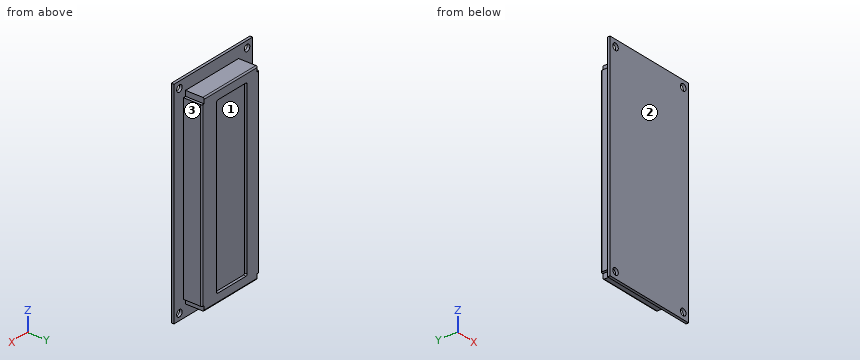
Autodesk Inventor part; units mm, degrees
ref_plane "YZ Plane" through (0, 0, 0) normal (1, 0, 0) x (0, 1, 0)
ref_plane "XZ Plane" through (0, 0, 0) normal (0, 1, 0) x (-1, 0, 0)
ref_plane "XY Plane" through (0, 0, 0) normal (0, 0, 1) x (1, 0, 0)
sketch "Sketch1" plane through (0, 0, 0) normal (0, 1, 0) x (-1, 0, 0)
  line L0 (-18, 40) -> (-18, -40)
  line L1 (-18, -40) -> (18, -40)
  line L2 (18, -40) -> (18, 40)
  line L3 (18, 40) -> (-18, 40)
  line L4 (-18, 40) -> (18, -40) construction
  line L5 (-18, -40) -> (18, 40) construction
  line L6 (18, 40) -> (-0.55, 40)
  line L7 (18, 40) -> (15.5, 40)
  line L8 (15.5, 40) -> (15.5, 37.5)
  circle A0 centre (15.5, 37.5) radius 1.25
  line L9 (15.5, 37.5) -> (-15.5, 37.5)
  line L10 (-15.5, 37.5) -> (-15.5, -37.5)
  line L11 (-15.5, -37.5) -> (15.5, -37.5)
  circle A1 centre (-15.5, 37.5) radius 1.25
  circle A2 centre (-15.5, -37.5) radius 1.25
  circle A3 centre (15.5, -37.5) radius 1.25
  point P0 (0, 0)
  dimension "d0" = 80
  dimension "d1" = 36
  dimension "d2" = 18.55
  dimension "d25" = 2.5
  dimension "d26" = 2.5
  dimension "d27" = 2.5
  dimension "d28" = 31
  dimension "d29" = 75
  dimension "d30" = 31
  dimension "d31" = 2.5
  dimension "d32" = 2.5
  dimension "d33" = 2.5
extrude "Extrusion1" add sketch "Sketch1" along normal blind 1 contours A3 | A2 L11 L10 | L10 L11 A2 | A1 L10 L9 | L9 L10 A1 | A0 L9 L8 | L8 L9 A0 | L3 L2 L1 L0
sketch "Sketch2" plane through (0, 1, 0) normal (0, 1, 0) x (1, 0, 0)
  line L0 (18, -40) -> (18, 40)
  line L1 (18, 40) -> (-18, 40)
  line L2 (-18, 40) -> (-18, -40)
  line L3 (-18, -40) -> (18, -40)
  line L4 (-18, -40) -> (0.55, -40)
  line L5 (-18, -40) -> (18, -40)
  line L6 (-11.6, -35.65) -> (-11.6, -33.65)
  line L7 (-11.6, -33.65) -> (-12.6, -33.65)
  line L8 (12.7, -35.65) -> (12.7, -33.65)
  line L9 (12.7, -33.65) -> (13.7, -33.65)
  line L10 (12.7, 35.65) -> (12.7, 33.65)
  line L11 (12.7, 33.65) -> (13.7, 33.65)
  line L12 (-11.6, 35.65) -> (-11.6, 33.65)
  line L13 (-11.6, 33.65) -> (-12.6, 33.65)
  line L14 (-11.6, -35.65) -> (12.7, -35.65)
  line L15 (13.7, -33.65) -> (13.7, 33.65)
  line L16 (12.7, 35.65) -> (-11.6, 35.65)
  line L17 (-12.6, 33.65) -> (-12.6, -33.65)
  point P0 (0, 0)
  dimension "d10" = 2
  dimension "d12" = 2
  dimension "d14" = 2
  dimension "d16" = 2
extrude "Extrusion2" add sketch "Sketch2" along normal blind 7 contours L6 L7 L17 L13 L12 L16 L10 L11 L15 L9 L8 L14
fillet "Fillet1" radius 0.5 4 edges at (-12.6, 8, 0) (0.55, 8, -35.65) (13.7, 8, 0) (0.55, 8, 35.65)
sketch "Sketch3" plane through (0, 8, 0) normal (0, 1, 0) x (1, 0, 0)
  line L0 (7, -32.25) -> (7, 32.25)
  line L1 (7, 32.25) -> (-7, 32.25)
  line L2 (-7, 32.25) -> (-7, -32.25)
  line L3 (-7, -32.25) -> (7, -32.25)
  line L4 (7, -32.25) -> (-7, 32.25) construction
  line L5 (7, 32.25) -> (-7, -32.25) construction
  point P0 (0, 0)
  dimension "d20" = 64.5
  dimension "d21" = 14
extrude "Extrusion3" cut sketch "Sketch3" against normal blind 1
fillet "Fillet2" radius 0.5 4 edges at (7, 7.5, -32.25) (7, 7.5, 32.25) (-7, 7.5, 32.25) (-7, 7.5, -32.25)
sketch "Sketch4" plane through (0, 1, 0) normal (0, 1, 0) x (1, 0, 0)
  line L0 (-18, 40) -> (-18, -40)
  line L1 (-18, -40) -> (18, -40)
  line L2 (18, -40) -> (18, 40)
  line L3 (18, 40) -> (-18, 40)
  line L4 (-18, 40) -> (18, -40) construction
  line L5 (-18, -40) -> (18, 40) construction
  line L6 (18, 40) -> (-0.55, 40)
  line L7 (18, 40) -> (15.5, 40)
  line L8 (15.5, 40) -> (15.5, 37.5)
  circle A0 centre (15.5, 37.5) radius 1.25
  line L9 (15.5, 37.5) -> (-15.5, 37.5)
  line L10 (-15.5, 37.5) -> (-15.5, -37.5)
  line L11 (-15.5, -37.5) -> (15.5, -37.5)
  circle A1 centre (-15.5, 37.5) radius 1.25
  circle A2 centre (-15.5, -37.5) radius 1.25
  circle A3 centre (15.5, -37.5) radius 1.25
  point P0 (0, 0)
  point P1 (0, 0)
  dimension "d34" = 80
  dimension "d35" = 36
  dimension "d36" = 18.55
  dimension "d37" = 2.5
  dimension "d38" = 2.5
  dimension "d39" = 2.5
  dimension "d40" = 31
  dimension "d41" = 75
  dimension "d42" = 31
  dimension "d43" = 2.5
  dimension "d44" = 2.5
  dimension "d45" = 2.5
extrude "Extrusion4" cut sketch "Sketch4" against normal blind 1 contours A3 | A2 L11 L10 | L10 L11 A2 | A1 L10 L9 | L9 L10 A1 | A0 L9 L8 | L8 L9 A0
properties part number "lcd05-16x2"
Part model, mm, in its own coordinate system. Face numbers are marked on the shaded views. Round coordinates to 2 decimals unless told otherwise and drop trailing zeros. Order: outer loops, then holes, each group sorted by start corner. A loop starts at its lowest first (then second) coordinate and runs counter-clockwise, first axis right, second up. Notation, with made-up numbers: M -24.5,39 L -3.5,39 A20 ccw -3.5,70 Z; hole C 16.5,66 d4. An arc over 180 degrees is marked long. Answer in a Markdown table with one row per item. Add a question column.
Q1. Cut at A-A on z = -37.5. Give the cut face in (x, y).
Q2. Cut at C-C on y = 2.25. Give the cut face in (x, z).
Q3. Pin check, flat tips, straight feed: pin 1 (2 mm diameter, centred on x = -3.5, y = 3, fed in from -Z); pin 2 (4 mm diameter, centred on y = 7, z = -27.5, fed in from -X); pin 3 (0.6 mm diameter, centred on y = 5.5, z = 35, fed in from -X). Stop position of each tip, or through.
Q4. Cut at B-B on x = -15.5. Give the cut face in (y, z), and give its area (3 significant figures).
Q5. Wall check: L1, parallel to Z at x = -15.5, y = 0.6; L2, parallel to X at y = 0.55, z = -37.5; L3, parallel to Y at x = 17, z = 23. Give the ranges that are in metal, low to high. Write a range as from..to.
Q6. Cut at D-D on x = -8. Give the cut face in (y, z).
Q7. Mould opens along X. For the marked faces 1, 2 and 3 say: +X half, -X half, draft (parallel to the pull), parting line (faces both ways), or undercut.
Established:
| question | item | result |
|---|---|---|
| 1 | outline | M -18,0 L -16.75,0 L -16.75,1 L -18,1 Z; M -14.25,0 L 14.25,0 L 14.25,1 L -14.25,1 Z; M 16.75,0 L 18,0 L 18,1 L 16.75,1 Z |
| 2 | outline | M -12.6,-33.65 L -11.6,-33.65 L -11.6,-35.65 L 12.7,-35.65 L 12.7,-33.65 L 13.7,-33.65 L 13.7,33.65 L 12.7,33.65 L 12.7,35.65 L -11.6,35.65 L -11.6,33.65 L -12.6,33.65 Z |
| 3 | pin 1 | stops at z = -35.65 |
| 3 | pin 2 | stops at x = -12.6 |
| 3 | pin 3 | stops at x = -11.6 |
| 4 | outline | M 0,-40 L 1,-40 L 1,-38.75 L 0,-38.75 Z; M 0,-36.25 L 1,-36.25 L 1,36.25 L 0,36.25 Z; M 0,38.75 L 1,38.75 L 1,40 L 0,40 Z |
| 4 | area | 75.0 mm2 |
| 5 | L1 | z = -40..-38.75, -36.25..36.25, 38.75..40 |
| 5 | L2 | x = -18..-16.75, -14.25..14.25, 16.75..18 |
| 5 | L3 | y = 0..1 |
| 6 | outline | M 0,-40 L 1,-40 L 1,-35.65 L 7.5,-35.65 A0.5 ccw 8,-35.15 L 8,35.15 A0.5 ccw 7.5,35.65 L 1,35.65 L 1,40 L 0,40 Z |
| 7 | face 1 | undercut |
| 7 | face 2 | draft |
| 7 | face 3 | +X half |
